The listing builds one solid part. Answer for the finished solid, in the listing's coordinates (mm). A direction names the side the tool comes from. Give positions to 0.01 mm unless a question says otherwise; leave off trailing zeros. Order: outer loops, then holes, each group sorted by start corner. A loop starts at its lowest first (then second) coordinate and runs counter-clockwise, first axis right, second up. Notation, with made-up numbers: (-32, 74.5) - (21, 74.5) arc R25 cw to (21, 88.5) - close; hole circle Ø2 at (24, 4.5). An arc over 180 degrees is marked (long way). Write each question's results on one line, items separated by ' | '. Start each with the question number.
1. Section A-A (x = 0) is taken. Give the vertices of the cut face in (y, z).
2. Which of the six approach directions +Z, -Z, +X, -X, +Y, -Y give full straight-line access (tool end or side, diameter ignored) to faces 4 (the face through (5, 7.144, 0)), 5 (the face through (-1.463, 1.274, -11.144))?
3. Section C-C (y = 6) is taken. Give the vertices of the cut face in (x, z) (1 decimal).
4. Section D-D (y = 1.25) is taken. Give the vertices of the cut face in (x, z) (1 decimal).
5. Find the intervals of material crossed by L1, parallel to X at y = 1, z = 0; L2, parallel to X at y = 3.5, z = 1.25, in increasing order.
6. Section B-B (z = 0) is taken. Give the vertices of the cut face in (x, y), and give its area (3 significant figures).
7. Flat-ended cylindrical pins translate along their axes: pin 1 (2 mm diameter, centred on x = -2.5, z = -1, fed in from +Y); pin 2 (1.5 mm diameter, centred on y = 5.5, z = -9, fed in from +X). Find the tip coordinate at first contact, or state that the pin passes through.
8. Determine the mould class of faces 1 (the face through (2.9, 3, -3.78)), 2 (the face through (-2.695, 5.695, 12.135)), 3 (the face through (11, 4.286, 5)) for opening direction X: released by +X, released by -X, zero draft, split by the parting line, or undercut.
from build123d import *

# Parameters (mm, degrees)
SKETCH2_R                = 11.1125
BOSS_EXTRUDE1_DEPTH      = 7.14375
SKETCH3_R                = 12.303125
BOSS_EXTRUDE2_DEPTH      = 1.5875
CUT_EXTRUDE2_DEPTH       = 19.808693033
CUT_EXTRUDE2_DEPTH_BACK  = 19.808693033
SKETCH4_R                = 4.7625
MOVE_FACE1_BY            = 1.27
MOVE_FACE1_2_BY          = 1.27
MOVE_START               = -1.27
MOVE_FACE2_OUTLINE_R     = 11.2395
MOVE_FACE2_OUTLINE_R_2   = 11.1125
MOVE_FACE2_DEPTH         = 5.55625
MOVE_START_2             = 4.28625
MOVE_FACE2_2_OUTLINE_R   = 12.430125
MOVE_FACE2_2_OUTLINE_R_2 = 12.303125
MOVE_FACE2_2_DEPTH       = 2.8575
CHAMFER1_SIZE            = 0.396875


# Read off the part's stored shape, not the designer's step: Move Face2
with BuildPart() as part:
    # Sketch2 → Boss-Extrude1 (new body)
    with BuildSketch(Plane(origin=(0, 0, 0), x_dir=(1, 0, 0), z_dir=(0, 1, 0))):
        with Locations(Location((0, 0, 0), (0, 0, 270))):
            Circle(SKETCH2_R)
    extrude(amount=BOSS_EXTRUDE1_DEPTH)

    # Sketch3 → Boss-Extrude2 (add)
    with BuildSketch(Plane(origin=(0, 7.14375, 0), x_dir=(1, 0, 0), z_dir=(0, 1, 0))):
        with Locations(Location((0, 0, 0), (0, 0, 270))):
            Circle(SKETCH3_R)
    extrude(amount=-BOSS_EXTRUDE2_DEPTH)

    # Sketch4 → Cut-Extrude2 (cut, two sides: drawn at the far end of the back side and taken through both)
    with BuildSketch(Plane(origin=(0, 0, 0), x_dir=(1, 0, 0), z_dir=(0, 1, 0)).offset(-CUT_EXTRUDE2_DEPTH_BACK)):
        with Locations(Location((0, 0, 0), (0, 0, 270))):
            Circle(SKETCH4_R)
    extrude(amount=CUT_EXTRUDE2_DEPTH + CUT_EXTRUDE2_DEPTH_BACK, mode=Mode.SUBTRACT)

    # Move Face1: a face moved outward by 1.27
    extrude(part.faces().sort_by_distance((-6.1515625, 5.55625, 9.8425))[0], amount=MOVE_FACE1_BY, dir=(0, -1, 0))

    # Move Face1 2: a face moved outward by 1.27
    extrude(part.faces().sort_by_distance((0, 0, 5.55625))[0], amount=MOVE_FACE1_2_BY, dir=(0, -1, 0))

    # Move Face2 outline → Move Face2 (add)
    with BuildSketch(Plane(origin=(0, 0, 0), x_dir=(1, 0, 0), z_dir=(0, 1, 0)).offset(MOVE_START)):
        Circle(MOVE_FACE2_OUTLINE_R)
        Circle(MOVE_FACE2_OUTLINE_R_2, mode=Mode.SUBTRACT)
    extrude(amount=MOVE_FACE2_DEPTH)

    # Move Face2 2 outline → Move Face2 2 (add)
    with BuildSketch(Plane(origin=(0, 0, 0), x_dir=(1, 0, 0), z_dir=(0, 1, 0)).offset(MOVE_START_2)):
        Circle(MOVE_FACE2_2_OUTLINE_R)
        Circle(MOVE_FACE2_2_OUTLINE_R_2, mode=Mode.SUBTRACT)
    extrude(amount=MOVE_FACE2_2_DEPTH)

    # Chamfer1
    chamfer1_edges = [part.edges().sort_by_distance(p)[0] for p in [
        (-11.2395, 4.28625, 0),
    ]]
    chamfer(chamfer1_edges, length=CHAMFER1_SIZE)


solid = part.part
Reported:
1) outline: (-1.27, -11.24) - (3.89, -11.24) - (4.29, -11.64) - (4.29, -12.43) - (7.14, -12.43) - (7.14, -4.76) - (-1.27, -4.76) - close; (-1.27, 4.76) - (7.14, 4.76) - (7.14, 12.43) - (4.29, 12.43) - (4.29, 11.64) - (3.89, 11.24) - (-1.27, 11.24) - close
2) face 4: +Z, -Z, +X, -X, +Y | face 5: -Y
3) outline: circle Ø24.9 at (0, 0); hole circle Ø9.5 at (0, 0)
4) outline: circle Ø22.5 at (0, 0); hole circle Ø9.5 at (0, 0)
5) L1: -11.24 to -4.76, 4.76 to 11.24 | L2: -11.17 to -4.6, 4.6 to 11.17
6) outline: (-12.43, 4.29) - (-11.64, 4.29) - (-11.24, 3.89) - (-11.24, -1.27) - (-4.76, -1.27) - (-4.76, 7.14) - (-12.43, 7.14) - close; (4.76, -1.27) - (11.24, -1.27) - (11.24, 3.89) - (11.64, 4.29) - (12.43, 4.29) - (12.43, 7.14) - (4.76, 7.14) - close | area: 116 mm²
7) pin 1: through | pin 2: x = 9.3
8) face 1: undercut | face 2: split by the parting line | face 3: zero draft
